For this review, take the finished solid that the model builds, in its own axes (mm). Face numbers are marked on the shaded views. A direction names the side the tool comes from. Coordinates: 2 decimals unless noted, no trailing zeros. Loops run counter-clockwise (first coordinate to the right, second up) from the corner with the lowest first, then second, coordinate; pieces in that order, holes last. Notation, with made-up numbers: M 84.25,2 L 92.25,2 A20 cw 92.25,6 Z; hole C 26.25,-38.75 d2. An arc over 180 degrees is marked long. Put each result on its own line as item: value.
```python
from build123d import *

# Parameters (mm, degrees)
BOSS_EXTRUDE1_DEPTH     = 12.7
CHAMFER1_SIZE           = 1.27
CUT_EXTRUDE1_DEPTH      = 3.175
F_8_CLEARANCE_HOLE1_D   = 4.9149
SKETCH5_W               = 11.3284
SKETCH5_H               = 7.9375
CUT_EXTRUDE_THIN1_DEPTH = 39.388001584
CHAMFER2_SIZE           = 2.54


with BuildPart() as part:
    # Sketch1 → Boss-Extrude1 (new body)
    with BuildSketch(Plane.XY):
        with BuildLine():
            Line((13.693796063, 21.648424474), (-13.693796063, 21.648424474))
            ThreePointArc((-13.693796063, 21.648424474), (0, -25.6159), (13.693796063, 21.648424474))
        make_face()
    extrude(amount=BOSS_EXTRUDE1_DEPTH)

    # Chamfer1
    chamfer1_edges = [part.edges().sort_by_distance(p)[0] for p in [
        (0, -25.6159, 12.7),
    ]]
    chamfer(chamfer1_edges, length=CHAMFER1_SIZE)

    # Sketch2 → Cut-Extrude1 (cut)
    with BuildSketch(Plane.XY.offset(12.7)):
        Polygon((-4.572, -2.639645431), (0, -5.279290861), (4.572, -2.639645431), (4.572, 2.639645431), (0, 5.279290861), (-4.572, 2.639645431), align=None)
    extrude(amount=-CUT_EXTRUDE1_DEPTH, mode=Mode.SUBTRACT)

    # #8 Clearance Hole1 (through all)
    with Locations(Plane.XY.offset(12.7)):
        with Locations((0, 0)):
            Hole(F_8_CLEARANCE_HOLE1_D / 2)

    # Sketch5 → Cut-Extrude-Thin1 (cut, through all)
    with BuildSketch(Plane.XY.offset(12.7)):
        Polygon((-7.405788321, -4.889701643), (-13.069988321, -14.700383827), (-6.195911679, -18.669133827), (-0.531711679, -8.858451643), align=None)
        with Locations((-13.6017, 0)):
            Rectangle(SKETCH5_W, SKETCH5_H)
        Polygon((-0.531711679, 8.858451643), (-6.195911679, 18.669133827), (-13.069988321, 14.700383827), (-7.405788321, 4.889701643), align=None)
        Polygon((7.405788321, 4.889701643), (13.069988321, 14.700383827), (6.195911679, 18.669133827), (0.531711679, 8.858451643), align=None)
        with Locations((13.6017, 0)):
            Rectangle(SKETCH5_W, SKETCH5_H)
        Polygon((0.531711679, -8.858451643), (6.195911679, -18.669133827), (13.069988321, -14.700383827), (7.405788321, -4.889701643), align=None)
    extrude(amount=-CUT_EXTRUDE_THIN1_DEPTH, mode=Mode.SUBTRACT)

    # Chamfer2
    chamfer2_edges = [part.edges().sort_by_distance(p)[0] for p in [
        (6.195911679, -18.669133827, 6.35),
        (0.531711679, -8.858451643, 6.35),
        (7.405788321, -4.889701643, 6.35),
        (13.069988321, -14.700383827, 6.35),
        (19.2659, -3.96875, 6.35),
        (7.9375, -3.96875, 6.35),
        (7.9375, 3.96875, 6.35),
        (19.2659, 3.96875, 6.35),
        (13.069988321, 14.700383827, 6.35),
        (7.405788321, 4.889701643, 6.35),
        (0.531711679, 8.858451643, 6.35),
        (6.195911679, 18.669133827, 6.35),
        (-6.195911679, 18.669133827, 6.35),
        (-0.531711679, 8.858451643, 6.35),
        (-7.405788321, 4.889701643, 6.35),
        (-13.069988321, 14.700383827, 6.35),
        (-19.2659, 3.96875, 6.35),
        (-7.9375, 3.96875, 6.35),
        (-7.9375, -3.96875, 6.35),
        (-19.2659, -3.96875, 6.35),
        (-13.069988321, -14.700383827, 6.35),
        (-7.405788321, -4.889701643, 6.35),
        (-0.531711679, -8.858451643, 6.35),
        (-6.195911679, -18.669133827, 6.35),
    ]]
    chamfer(chamfer2_edges, length=CHAMFER2_SIZE)


solid = part.part
```
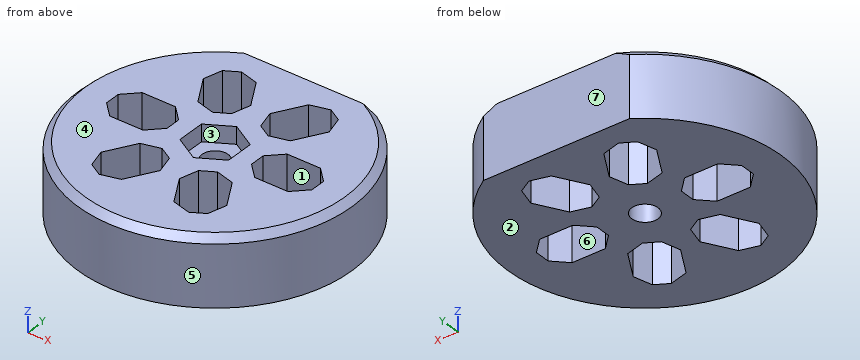
(1) Add section A-A (y = 0). Write out the cut boundary in (x, z) (1 decimal), plus the area to 3 significant figures.
Determined:
outline: M -25.6,0 L -19.3,0 L -19.3,12.7 L -24.3,12.7 L -25.6,11.4 Z; M -7.9,0 L -2.5,0 L -2.5,9.5 L -4.6,9.5 L -4.6,12.7 L -7.9,12.7 Z; M 2.5,0 L 7.9,0 L 7.9,12.7 L 4.6,12.7 L 4.6,9.5 L 2.5,9.5 Z; M 19.3,0 L 25.6,0 L 25.6,11.4 L 24.3,12.7 L 19.3,12.7 Z
area: 285 mm^2
(2) Draft analysis for pull direction Y (two halves, no side actions). For the marked faces 4, 5, 6 and 7, state which applies: +Y half, -Y half, draft (parallel to the pull), parting line (faces both ways), or undercut.
Determined:
face 4: draft
face 5: parting line
face 6: undercut
face 7: +Y half
(3) Tool access review of the marked faces 1, 2 and 3: name each direction out of +Z, -Z, +X, -X, +Y, -Y from which nothing blocks a thin tool from reaching the whole face with its end or side.
Determined:
face 1: +Z, -Z
face 2: -Z, +X, -X, +Y, -Y
face 3: +Z
(4) Wall thickness on line 1 along Y through (x, z) = (-8.5, 1); line 2 along Y through (x, z) = (8, 9); line 3 along X through (y, z) = (10.5, 10): over which ranges is each line inside the solid? List them lowest first. Write a range as [from, to].
Determined:
line 1: y = [-24.16, -17.34], [-7.04, -1.99], [1.99, 7.04], [17.34, 21.65]
line 2: y = [-24.33, -17.29], [-6.91, -1.49], [1.49, 6.91], [17.29, 21.65]
line 3: x = [-23.37, -10.64], [-1.95, 1.95], [10.64, 23.37]
(5) For pin 1 (0.9 mm diameter, centred on y = -0.5, z = 4, fed in from +X); pin 2 (1 mm diameter, centred on y = -20.5, z = 4, fed in from +X); pin 3 (2 mm diameter, centred on x = -10.5, z = 3, fed in from -Y); pin 4 (2 mm diameter, centred on x = 12, z = 7.5, fed in from -Y), all flat-tipped, find the tip position at first contact; note any pin that passes through.
Determined:
pin 1: stops at x = 25.62
pin 2: stops at x = 16.01
pin 3: stops at y = -23.79
pin 4: stops at y = -23.13
(6) Add section B-B (z = 5.5). State how many separate pieces and enclosed holes the cut face has, plus the area to 3 significant figures.
Determined:
separate pieces: 1
enclosed holes: 7
area: 1,510 mm^2
